Geometry check sheet. Reference: the model listing, model coordinates, mm. Face numbers are marked on the shaded views. Give positions to 0.01 mm unless a question says otherwise; leave off trailing zeros. Order: outer loops, then holes, each group sorted by start corner. A loop starts at its lowest first (then second) coordinate and runs counter-clockwise, first axis right, second up.
```python
from build123d import *

# Parameters (mm, degrees)
SKETCH1_R           = 127
BOSS_EXTRUDE1_DEPTH = 76.2
SKETCH2_R           = 88.9
BOSS_EXTRUDE2_DEPTH = 25.4
SKETCH3_R           = 12.7
BOSS_EXTRUDE3_DEPTH = 50.8
SKETCH4_R           = 88.9
BOSS_EXTRUDE4_DEPTH = 25.4
SKETCH6_R           = 12.7
BOSS_EXTRUDE5_DEPTH = 812.8
SKETCH7_R           = 88.9
BOSS_EXTRUDE6_DEPTH = 25.4
SKETCH8_R           = 127
BOSS_EXTRUDE7_DEPTH = 76.2
SKETCH9_R           = 88.9
BOSS_EXTRUDE8_DEPTH = 25.4
SKETCH10_R          = 12.7
BOSS_EXTRUDE9_DEPTH = 50.8


with BuildPart() as part:
    # Sketch1 → Boss-Extrude1 (new body)
    with BuildSketch(Plane.XY):
        Circle(SKETCH1_R)
    extrude(amount=-BOSS_EXTRUDE1_DEPTH)

    # Sketch2 → Boss-Extrude2 (add)
    with BuildSketch(Plane.XY):
        Circle(SKETCH2_R)
    extrude(amount=BOSS_EXTRUDE2_DEPTH)

    # Sketch3 → Boss-Extrude3 (add)
    with BuildSketch(Plane.XY.offset(25.4)):
        Circle(SKETCH3_R)
    extrude(amount=BOSS_EXTRUDE3_DEPTH)

    # Sketch4 → Boss-Extrude4 (add)
    with BuildSketch(Plane(origin=(0, 0, -76.2), x_dir=(-1, 0, 0), z_dir=(0, 0, -1))):
        Circle(SKETCH4_R)
    extrude(amount=BOSS_EXTRUDE4_DEPTH)

    # Sketch6 → Boss-Extrude5 (add)
    with BuildSketch(Plane(origin=(0, 0, -101.6), x_dir=(-1, 0, 0), z_dir=(0, 0, -1))):
        Circle(SKETCH6_R)
    extrude(amount=BOSS_EXTRUDE5_DEPTH)

    # Sketch7 → Boss-Extrude6 (add)
    with BuildSketch(Plane(origin=(0, 0, -914.4), x_dir=(-1, 0, 0), z_dir=(0, 0, -1))):
        Circle(SKETCH7_R)
    extrude(amount=BOSS_EXTRUDE6_DEPTH)

    # Sketch8 → Boss-Extrude7 (add)
    with BuildSketch(Plane(origin=(0, 0, -939.8), x_dir=(-1, 0, 0), z_dir=(0, 0, -1))):
        Circle(SKETCH8_R)
    extrude(amount=BOSS_EXTRUDE7_DEPTH)

    # Sketch9 → Boss-Extrude8 (add)
    with BuildSketch(Plane(origin=(0, 0, -1016), x_dir=(-1, 0, 0), z_dir=(0, 0, -1))):
        Circle(SKETCH9_R)
    extrude(amount=BOSS_EXTRUDE8_DEPTH)

    # Sketch10 → Boss-Extrude9 (add)
    with BuildSketch(Plane(origin=(0, 0, -1041.4), x_dir=(-1, 0, 0), z_dir=(0, 0, -1))):
        Circle(SKETCH10_R)
    extrude(amount=BOSS_EXTRUDE9_DEPTH)


solid = part.part
```
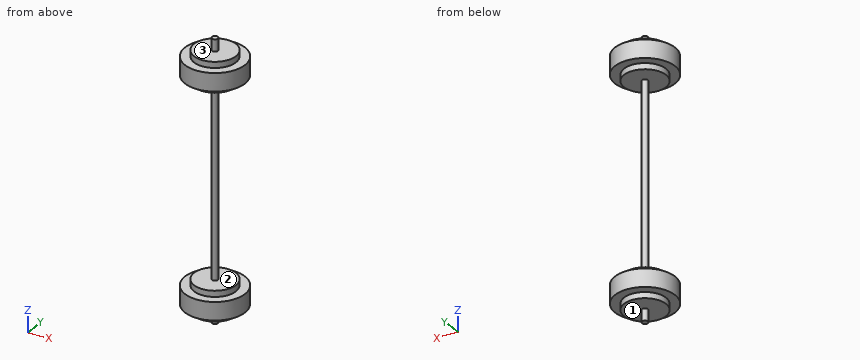
Q1. Cross-section at A-A, the plane y = -53.5. Record the boundary of the cut face in (x, z).
Q2. Release check for a two-part mould opening along Z. For the marked faces 1, 2 and 3 record: pulls with the +Z half, pulls with the -Z half, needs draft (parallel to the pull), parting line crosses it, or undercut.
Q3. Gauge pin test, flat ends, axial feed: P1, Ø12, axis at x = 11.5, z = -110.5, coming from the +Y side; P2, Ø12, axis at y = -0.5, z = -839, coming from the -X side; P3, Ø12, axis at y = -16.5, z = -422.5, coming from the +X side. Record the tip position at first contact, or that the pin passes through.
Q4. Cross-section at D-D, the plane z = -89. Record the boundary of the cut face in (x, y).
Q5. Thickness scan on L1, parallel to Z at x = -7, y = 39; L2, parallel to Z at x = 86, y = 68; L3, parallel to X at y = -2, z = -465. Record the ranges inside material, lowest first.
Q6. Cross-section at C-C, the plane y = 106. Record the boundary of the cut face in (x, z).
Q7. Cross-section at B-B, the plane z = -737. Record the boundary of the cut face in (x, y), and give its area (3 significant figures).
Answers follow:
1. outline: (-115.18, -1016) - (-71, -1016) - (-71, -1041.4) - (71, -1041.4) - (71, -1016) - (115.18, -1016) - (115.18, -939.8) - (71, -939.8) - (71, -914.4) - (-71, -914.4) - (-71, -939.8) - (-115.18, -939.8) - close; (-115.18, -76.2) - (-71, -76.2) - (-71, -101.6) - (71, -101.6) - (71, -76.2) - (115.18, -76.2) - (115.18, 0) - (71, 0) - (71, 25.4) - (-71, 25.4) - (-71, 0) - (-115.18, 0) - close
2. face 1: pulls with the -Z half
2. face 2: undercut
2. face 3: pulls with the +Z half
3. P1: stops at y = 11.45
3. P2: stops at x = -12.7
3. P3: stops at x = 7.14
4. outline: circle Ø177.8 at (0, 0)
5. L1: z = -1041.4 to -914.4, -101.6 to 25.4
5. L2: z = -1016 to -939.8, -76.2 to 0
5. L3: x = -12.54 to 12.54
6. outline: (-69.95, -1016) - (69.95, -1016) - (69.95, -939.8) - (-69.95, -939.8) - close; (-69.95, -76.2) - (69.95, -76.2) - (69.95, 0) - (-69.95, 0) - close
7. outline: circle Ø25.4 at (0, 0)
7. area: 507 mm2
